Build history of the part. All positions in model axes, mm. A direction names the side the tool comes from. Give positions to 0.01 mm unless a question says otherwise; leave off trailing zeros. Order: outer loops, then holes, each group sorted by start corner. A loop starts at its lowest first (then second) coordinate and runs counter-clockwise, first axis right, second up. Notation, with made-up numbers: (27, -3) - (52, -3) arc R37 ccw to (52, 35) - close; hole circle Ø6 at (47, 51). An arc over 180 degrees is marked (long way). Write each question's results on one line, items separated by ' | '. Start each with the question number.
from build123d import *

# Parameters (mm, degrees)
F0_R      = 7.8435703096
F1_DEPTH  = 5.67
F0_R_2    = 7.7757185056
F2_W      = 17.6903378959
F2_H      = 15.67
F3_DEPTH  = 5.67
F4_R      = 1.425
F5_DEPTH  = 10.38
F6_R      = 1.425
F7_DEPTH  = 10.38
F8_R      = 2.465
F9_DEPTH  = 2.425
F10_W     = 12.8629952669
F10_H     = 10.9573621303
F11_DEPTH = 3
F12_R     = 2.75
F12_R_2   = 1.75
F13_DEPTH = 2
F14_R     = 4.345
F14_R_2   = 3.4662678384
F15_DEPTH = 25
F14_R_3   = 3.1273613379
F14_R_4   = 4.1038801884
F14_R_5   = 4.2870364602
F16_DEPTH = 25


with BuildPart() as f1:
    # F0 (on Front) → F1 (new body)
    with BuildSketch(Plane.XZ):
        with Locations((-31.0182443455, 13.5022135742)):
            Circle(F0_R)
    extrude(amount=F1_DEPTH)

    # F14 (on Front) → F15, piece 2 (join)
    with BuildSketch(Plane.XZ):
        with Locations((-31.2459040433, 14.0220327303)):
            Circle(F14_R)
        with Locations((-31.2459040433, 14.0220327303)):
            Circle(F14_R_3, mode=Mode.SUBTRACT)
    extrude(amount=F15_DEPTH)

    # F14 (on Front) → F16 (cut)
    with BuildSketch(Plane.XZ):
        with Locations((27.6749636978, 13.738758862)):
            Circle(F14_R)
        with Locations((27.6749636978, 13.738758862)):
            Circle(F14_R_2, mode=Mode.SUBTRACT)
        with Locations((-30.9626311064, -35.5508103967)):
            Circle(F14_R)
        with Locations((-30.9626311064, -35.5508103967)):
            Circle(F14_R_4, mode=Mode.SUBTRACT)
        with Locations((27.9582366347, -35.5508103967)):
            Circle(F14_R)
        with Locations((27.9582366347, -35.5508103967)):
            Circle(F14_R_5, mode=Mode.SUBTRACT)
        with Locations((-31.2459040433, 14.0220327303)):
            Circle(F14_R)
        with Locations((-31.2459040433, 14.0220327303)):
            Circle(F14_R_3, mode=Mode.SUBTRACT)
    extrude(amount=-F16_DEPTH, mode=Mode.SUBTRACT)


with BuildPart() as f1b:
    # F0 (on Front) → F1, piece 2 (new body)
    with BuildSketch(Plane.XZ):
        with Locations((27.6562659057, 13.5022135742)):
            Circle(F0_R_2)
    extrude(amount=F1_DEPTH)

    # F14 (on Front) → F15 (join)
    with BuildSketch(Plane.XZ):
        with Locations((27.6749636978, 13.738758862)):
            Circle(F14_R)
        with Locations((27.6749636978, 13.738758862)):
            Circle(F14_R_2, mode=Mode.SUBTRACT)
    extrude(amount=F15_DEPTH)


with BuildPart() as f1c:
    # F0 (on Front) → F1, piece 3 (new body)
    with BuildSketch(Plane.XZ):
        with Locations((-31.0182443455, -35.7866174178)):
            Circle(F0_R_2)
    extrude(amount=F1_DEPTH)

    # F14 (on Front) → F15, piece 3 (join)
    with BuildSketch(Plane.XZ):
        with Locations((-30.9626311064, -35.5508103967)):
            Circle(F14_R)
        with Locations((-30.9626311064, -35.5508103967)):
            Circle(F14_R_4, mode=Mode.SUBTRACT)
    extrude(amount=F15_DEPTH)


with BuildPart() as f1d:
    # F0 (on Front) → F1, piece 4 (new body)
    with BuildSketch(Plane.XZ):
        with Locations((27.6562659057, -35.7866174178)):
            Circle(F0_R_2)
    extrude(amount=F1_DEPTH)

    # F14 (on Front) → F15, piece 4 (join)
    with BuildSketch(Plane.XZ):
        with Locations((27.9582366347, -35.5508103967)):
            Circle(F14_R)
        with Locations((27.9582366347, -35.5508103967)):
            Circle(F14_R_5, mode=Mode.SUBTRACT)
    extrude(amount=F15_DEPTH)


with BuildPart() as f3:
    # F2 (on Front) → F3 (new body)
    with BuildSketch(Plane.XZ):
        with Locations((-76.0589055717, 37.1088152751)):
            Rectangle(F2_W, F2_H)
    extrude(amount=F3_DEPTH)

    # F4 (on face) → F5 (join)
    with BuildSketch(Plane(origin=(-84.9040745196, 0, 0), x_dir=(0, -1, 0), z_dir=(-1, 0, 0))):
        with Locations((2.974371193, 37.1088152751)):
            Circle(F4_R)
    extrude(amount=F5_DEPTH)

    # F6 (on face) → F7 (join)
    with BuildSketch(Plane.YZ.offset(-67.2137366238)):
        with Locations((-3.0722431839, 37.1088152751)):
            Circle(F6_R)
    extrude(amount=F7_DEPTH)

    # F8 (on face) → F9 (join)
    with BuildSketch(Plane.XZ.offset(5.67)):
        with Locations((-80.3711495243, 41.4787063429)):
            Circle(F8_R)
        with Locations((-72.1980867, 41.4787063429)):
            Circle(F8_R)
        with Locations((-72.1980867, 33.8693021292)):
            Circle(F8_R)
        with Locations((-80.3711495243, 33.8693021292)):
            Circle(F8_R)
    extrude(amount=F9_DEPTH)

    # F10 (on face) → F11 (cut)
    with BuildSketch(Plane(origin=(0, 0, 0), x_dir=(-1, 0, 0), z_dir=(0, 1, 0))):
        with Locations((76.6844823956, 36.675314419)):
            Rectangle(F10_W, F10_H)
    extrude(amount=-F11_DEPTH, mode=Mode.SUBTRACT)

    # F12 (on face) → F13 (join)
    with BuildSketch(Plane(origin=(0, -3, 0), x_dir=(-1, 0, 0), z_dir=(0, 1, 0))):
        with Locations((76.6844823956, 36.5562103689)):
            Circle(F12_R)
        with Locations((76.6844823956, 36.5562103689)):
            Circle(F12_R_2, mode=Mode.SUBTRACT)
    extrude(amount=F13_DEPTH)


solid = f3.part
Item 1: Probe line 1 along X through (y, z) = (-2.25, 40.25); line 2 along X through (y, z) = (-4.5, 35); line 3 along Z through (x, y) = (-60, -3). List the from-to ranges inside material, lowest first. Write a range as from..to.
Item 2: Cut at B-B, the plane z = 32.75. List the corners of the cut face in (x, y) (3 decimals), then the cut area to 3 significant figures.
Item 3: Cut at A-A, the plane y = -2. List the corners of the cut face in (x, z), then the cut area to 3 significant figures.
Item 4: Cut at D-D, the plane y = -6.5. List the corners of the cut face in (x, z) (3 decimals), then the cut area to 3 significant figures.
Item 5: Flat gauge pins, fed straight in: pin 1 Ø1.8 at (x, z) = (-76, 37) entering from +Y; pin 2 Ø5.5 at (x, z) = (-74.5, 35.5) entering from +Y; pin 3 Ø3 at (x, z) = (-84.5, 42) entering from -Y. Where does each tip first touch, or does it go through?
Item 6: Cut at C-C, the plane x = -79. List the corners of the cut face in (y, z) (3 decimals), then the cut area to 3 significant figures.
Item 7: Two-plate mould, pull along X, no slides. Class faces 1 (the flat face through (-80, -8.095, 42)), 2 (the flat face through (-84.904, -3, 39)), 3 (the flat face through (-77, -1, 31.197)): +X half, -X half, draft (parallel to the pull), parting line (faces both ways), or undercut.
Item 8: Which spindle directions (+Z, -Z, +X, -X, +Y, -Y) get a long thin tool onto all of the face, cutting with end or side? Do faces 4 (the cylindrical face through (-74.015, -6.866, 43.145)), 5 (the flat face through (-78, -3, 39.2)), 6 (the cylindrical face through (-90.021, -3.632, 35.845)). Say none if no direction does.
Values found:
1) line 1: x = -84.9..-83.12, -70.25..-67.21 | line 2: x = -84.9..-67.21 | line 3: z = 35.69..38.53
2) outline: (-84.904, -5.67) - (-82.567, -5.67) - (-82.567, -8.095) - (-78.175, -8.095) - (-78.175, -5.67) - (-74.394, -5.67) - (-74.394, -8.095) - (-70.002, -8.095) - (-70.002, -5.67) - (-67.214, -5.67) - (-67.214, 0) - (-70.253, 0) - (-70.253, -3) - (-83.116, -3) - (-83.116, 0) - (-84.904, 0) - close | area: 83.0 mm2
3) outline: (-95.28, 36.07) - (-84.9, 36.07) - (-84.9, 29.27) - (-67.21, 29.27) - (-67.21, 36.17) - (-56.83, 36.17) - (-56.83, 38.05) - (-67.21, 38.05) - (-67.21, 44.94) - (-84.9, 44.94) - (-84.9, 38.15) - (-95.28, 38.15) - close; circle Ø5.5 at (-76.68, 36.56); hole (-83.12, 31.2) - (-70.25, 31.2) - (-70.25, 42.15) - (-83.12, 42.15) - close; hole circle Ø3.5 at (-76.68, 36.56) | area: 191 mm2
4) outline: circle Ø4.93 at (-80.371, 33.869); circle Ø4.93 at (-80.371, 41.479); circle Ø4.93 at (-72.198, 33.869); circle Ø4.93 at (-72.198, 41.479) | area: 76.4 mm2
5) pin 1: stops at y = -3 | pin 2: stops at y = -1 | pin 3: stops at y = -5.67
6) outline: (-8.095, 31.821) - (-5.67, 31.821) - (-5.67, 29.274) - (0, 29.274) - (0, 31.197) - (-3, 31.197) - (-3, 35.073) - (-1, 35.073) - (-1, 38.04) - (-3, 38.04) - (-3, 42.154) - (0, 42.154) - (0, 44.944) - (-5.67, 44.944) - (-5.67, 43.527) - (-8.095, 43.527) - (-8.095, 39.43) - (-5.67, 39.43) - (-5.67, 35.918) - (-8.095, 35.918) - close | area: 81.8 mm2
7) face 1: draft | face 2: -X half | face 3: undercut
8) face 4: -Y | face 5: +Y | face 6: -X
